CAD build for the part. Positions are in the model's coordinates, mm. A direction names the side the tool comes from. Give positions to 0.01 mm unless a question says otherwise; leave off trailing zeros. Order: outer loops, then holes, each group sorted by start corner. A loop starts at its lowest first (then second) coordinate and runs counter-clockwise, first axis right, second up. Notation, with made-up numbers: (78.5, -4.75) -> (84.5, -4.75) arc R14 cw to (84.5, 8.25) -> close; hole circle Ø10 at (64, -39). An arc over 180 degrees is marked (long way). Answer as CSV lines item,"result".
```python
from build123d import *

# Parameters (mm, degrees)
F0_W        = 20
F0_H        = 20
F1_DEPTH    = 5
F2_W        = 3.5
F2_H        = 16.5
F3_DEPTH    = 1.2
F4_R        = 4
F5_DEPTH    = 5.001
F6_R        = 2
F7_W        = 0.6
F7_H        = 3.8
F8_DEPTH    = 2.5
F9_T1_DEPTH = 3.8
F9_T3_DEPTH = 5.8


# Not quite as in the source:
# - a fillet or chamfer that OpenCascade refuses, or shapes differently, is made with other operations: its cross-section is extruded or revolved along the edge and cut away or added


with BuildPart() as f1:
    # F0 (on Top) → F1 (new body)
    with BuildSketch(Plane.XY):
        Rectangle(F0_W, F0_H)
    extrude(amount=F1_DEPTH)

    # F2 (on face) → F3 (cut)
    with BuildSketch(Plane(origin=(0, 0, 0), x_dir=(1, 0, 0), z_dir=(0, 0, -1))):
        with Locations((-8.25, -1.75)):
            Rectangle(F2_W, F2_H)
    extrude(amount=-F3_DEPTH, mode=Mode.SUBTRACT)

    # F4 (on face) → F5 (cut, through all)
    with BuildSketch(Plane.XY.offset(5)):
        with Locations((2, -2)):
            Circle(F4_R)
    extrude(amount=-F5_DEPTH, mode=Mode.SUBTRACT)

    # F6
    f6_edges = [f1.edges().sort_by_distance(p)[0] for p in [
        (10, -10, 2.5),
        (-10, -10, 2.5),
        (-10, 10, 3.1),
        (10, 10, 2.5),
    ]]
    fillet(f6_edges, radius=F6_R)

    # F7 (on face) → F8 (cut)
    with BuildSketch(Plane(origin=(-10, 0, 0), x_dir=(0, -1, 0), z_dir=(-1, 0, 0))):
        with Locations((-2.3, 3.1)):
            Rectangle(F7_W, F7_H)
        with Locations((2.3, 3.1)):
            Rectangle(F7_W, F7_H)
    extrude(amount=-F8_DEPTH, mode=Mode.SUBTRACT)

    # F9: fillet of radius 0.4 on 8 edges, made by hand

    # F9_s2 → F9_t1 (join)
    with BuildSketch(Plane.XY.offset(1.2)):
        with BuildLine():
            ThreePointArc((-7.5, 2.2), (-7.6171572875, 2.4828427125), (-7.9, 2.6))
            Line((-7.9, 2.6), (-7.5, 2.6))
            Line((-7.5, 2.6), (-7.5, 2.2))
        make_face()
        with BuildLine():
            ThreePointArc((-7.9, 2), (-7.6171572875, 2.1171572875), (-7.5, 2.4))
            Line((-7.5, 2.4), (-7.5, 2))
            Line((-7.5, 2), (-7.9, 2))
        make_face()
        with BuildLine():
            ThreePointArc((-7.9, -2.6), (-7.6171572875, -2.4828427125), (-7.5, -2.2))
            Line((-7.5, -2.2), (-7.5, -2.6))
            Line((-7.5, -2.6), (-7.9, -2.6))
        make_face()
        with BuildLine():
            ThreePointArc((-7.5, -2.4), (-7.6171572875, -2.1171572875), (-7.9, -2))
            Line((-7.9, -2), (-7.5, -2))
            Line((-7.5, -2), (-7.5, -2.4))
        make_face()
    extrude(amount=F9_T1_DEPTH)

    # F9_s4 → F9_t3 (cut)
    with BuildSketch(Plane.XY.offset(0.2)):
        with BuildLine():
            ThreePointArc((-10, 1.6), (-9.8828427125, 1.8828427125), (-9.6, 2))
            Line((-9.6, 2), (-10, 2))
            Line((-10, 2), (-10, 1.6))
        make_face()
        with BuildLine():
            ThreePointArc((-9.6, -2), (-9.8828427125, -1.8828427125), (-10, -1.6))
            Line((-10, -1.6), (-10, -2))
            Line((-10, -2), (-9.6, -2))
        make_face()
        with BuildLine():
            ThreePointArc((-10, -3), (-9.8828427125, -2.7171572875), (-9.6, -2.6))
            Line((-9.6, -2.6), (-10, -2.6))
            Line((-10, -2.6), (-10, -3))
        make_face()
        with BuildLine():
            ThreePointArc((-9.6, 2.6), (-9.8828427125, 2.7171572875), (-10, 3))
            Line((-10, 3), (-10, 2.6))
            Line((-10, 2.6), (-9.6, 2.6))
        make_face()
    extrude(amount=F9_T3_DEPTH, mode=Mode.SUBTRACT)


solid = f1.part
```
1) Pin check, flat tips, straight feed: P1, Ø1.4, axis at x = -9, z = 3, coming from the -Y side; P2, Ø1.3, axis at x = -9, z = 0.5, coming from the +Y side; P3, Ø0.5, axis at x = -9, z = 2.5, coming from the +Y side. Stop position of each tip, or through.
Data:
P1,"stops at y = -9.98"
P2,"stops at y = -6.5"
P3,"stops at y = 9.85"
2) Which spindle directions (+Z, -Z, +X, -X, +Y, -Y) get a long thin tool onto all of the face, cutting with end or side? Do faces 4 (the flat face through (-9, -2, 3)), 5 (the flat face through (-10, -6, 3)). Say none if no direction does.
Data:
face 4,"+Z, -Z, -X"
face 5,"+Z, -Z, -X, +Y, -Y"
3) Band-saw the part on C-C, the plane z = 2.2. Write the cut outline in (x, y), then the cut area to 3 significant figures.
Data:
outline,"(-10, -8) arc R2 ccw to (-8, -10) -> (8, -10) arc R2 ccw to (10, -8) -> (10, 8) arc R2 ccw to (8, 10) -> (-8, 10) arc R2 ccw to (-10, 8) -> (-10, 3) arc R0.4 ccw to (-9.6, 2.6) -> (-7.9, 2.6) arc R0.4 cw to (-7.51, 2.3) arc R0.4 cw to (-7.9, 2) -> (-9.6, 2) arc R0.4 ccw to (-10, 1.6) -> (-10, -1.6) arc R0.4 ccw to (-9.6, -2) -> (-7.9, -2) arc R0.4 cw to (-7.51, -2.3) arc R0.4 cw to (-7.9, -2.6) -> (-9.6, -2.6) arc R0.4 ccw to (-10, -3) -> close; hole circle Ø8 at (2, -2)"
area,"343 mm2"
4) Band-saw the part on D-D, the plane x = -8.25. Write the cut outline in (y, z), then the cut area to 3 significant figures.
Data:
outline,"(-9.98, 0) -> (-6.5, 0) -> (-6.5, 1.2) -> (-2.6, 1.2) -> (-2.6, 5) -> (-9.98, 5) -> close; (-2, 1.2) -> (2, 1.2) -> (2, 5) -> (-2, 5) -> close; (2.6, 1.2) -> (9.98, 1.2) -> (9.98, 5) -> (2.6, 5) -> close"
area,"75.5 mm2"
5) Band-saw the part on B-B, the plane y = 0. Write the cut outline in (x, z), then the cut area to 3 significant figures.
Data:
outline,"(-10, 1.2) -> (-6.5, 1.2) -> (-6.5, 0) -> (-1.46, 0) -> (-1.46, 5) -> (-10, 5) -> close; (5.46, 0) -> (10, 0) -> (10, 5) -> (5.46, 5) -> close"
area,"61.2 mm2"
6) Band-saw the part on A-A, the plane x = 2. Write the cut outline in (y, z), then the cut area to 3 significant figures.
Data:
outline,"(-10, 0) -> (-6, 0) -> (-6, 5) -> (-10, 5) -> close; (2, 0) -> (10, 0) -> (10, 5) -> (2, 5) -> close"
area,"60.0 mm2"
7) Pull direction Y, two halves, no side cores. Call faces 1 (the flat face through (-9, 2, 3)), 2 (the flat face through (-8, -6.5, 1)), 3 (the flat face through (-6.5, 2, 1)): pulls with the +Y half, pulls with the -Y half, needs draft (parallel to the pull), parting line crosses it, or undercut.
Data:
face 1,"undercut"
face 2,"pulls with the +Y half"
face 3,"needs draft"
8) Wall check: line 1 along Y through (x, z) = (2, 2.7); line 2 along Y through (x, z) = (-8, 1.5); line 3 along Z through (x, y) = (-8.75, -3.5). Give the ranges that are in metal, low to high. Write a range as [from, to].
Data:
line 1,"y = [-10, -6], [2, 10]"
line 2,"y = [-10, -2.6], [-2, 2], [2.6, 10]"
line 3,"z = [1.2, 5]"
